Verification items for the finished model (mm, model axes). A direction names the side the tool comes from. Give positions to 0.01 mm unless a question says otherwise; leave off trailing zeros. Loops run counter-clockwise (first coordinate to the right, second up) from the corner with the lowest first, then second, coordinate; pieces in that order, holes last. Notation, with made-up numbers: M -27,-19 L 4,-19 A14 cw 4,1 Z; hole C -5,-8 d1. An arc over 180 degrees is marked long. Use a Markdown table: item, result.
from build123d import *

# Parameters (mm, degrees)
F1_DEPTH = 62.4
F4_DEPTH = 24.5
F5_W     = 19.0535837948
F5_H     = 11.2809054554
F5_H_2   = 2.8878487647
F6_DEPTH = 4.1


# Not quite as in the source:
# - a pattern or mirror of a feature is missing from the dataset's text; its kind, count and spacing are read off the source's solid


with BuildPart() as f1:
    # F0 (on Right) → F1 (new body)
    with BuildSketch(Plane.YZ):
        Polygon((24.6393419802, 87.7444967628), (5.7596671395, 54.6524040401), (5.7596671395, 37.0838306844), (49.7630737395, 15.9439614351), (358.1593094913, 15.9439614351), (388.9961540699, 31.0895591974), (388.9961540699, 87.2576609254), (339.3792808056, 93.3623313904), (64.8232772946, 93.3623313904), align=None)
    extrude(amount=F1_DEPTH)

    # F2: F1 across plane


with BuildPart() as f1_1:
    add(f1.part)
    add(f1.part.mirror(Plane.YZ))

    # F3 (on face) → F4 (cut)
    with BuildSketch(Plane.YZ.offset(62.4)):
        Polygon((59.2419728637, 15.9439614351), (127.3969262838, 15.9439614351), (127.3969262838, 41.5049567819), (110.9381020069, 60.795918107), (75.7007971406, 60.795918107), (59.2419728637, 41.5049567819), align=None)
        Polygon((230.519130826, 15.9439614351), (342.7896499634, 15.9439614351), (342.7896499634, 36.7200672626), (333.9802026749, 60.795918107), (241.1305308342, 60.795918107), (230.519130826, 41.8756008148), align=None)
    f4 = extrude(amount=-F4_DEPTH, mode=Mode.SUBTRACT)

    # F4_copies: F4 across plane
    add(f4.mirror(Plane(origin=(0, 0, 0), x_dir=(0, 0, -1), z_dir=(-1, 0, 0))), mode=Mode.SUBTRACT)

    # F5 (on face) → F6 (cut)
    with BuildSketch(Plane.XZ.offset(-5.7596671395)):
        with Locations((52.8732081026, 42.7242834121)):
            Rectangle(F5_W, F5_H)
        with Locations((52.8732081026, 35.6399063021)):
            Rectangle(F5_W, F5_H_2)
    f6 = extrude(amount=-F6_DEPTH, mode=Mode.SUBTRACT)

    # F6_copies: F6 across plane
    add(f6.mirror(Plane(origin=(0, 0, 0), x_dir=(0, 0, -1), z_dir=(-1, 0, 0))), mode=Mode.SUBTRACT)


solid = f1_1.part
(1) Cross-section at C-C on x = 51. Record the cut outline in (y, z).
Results below:
| item | result |
|---|---|
| outline | M 5.76,48.36 L 9.86,48.36 L 9.86,35.11 L 49.76,15.94 L 59.24,15.94 L 59.24,41.5 L 75.7,60.8 L 110.94,60.8 L 127.4,41.5 L 127.4,15.94 L 230.52,15.94 L 230.52,41.88 L 241.13,60.8 L 333.98,60.8 L 342.79,36.72 L 342.79,15.94 L 358.16,15.94 L 389,31.09 L 389,87.26 L 339.38,93.36 L 64.82,93.36 L 24.64,87.74 L 5.76,54.65 Z |
(2) Cross-section at A-A on y = 310.5. Record the cut outline in (x, z).
Results below:
| item | result |
|---|---|
| outline | M -62.4,60.8 L -37.9,60.8 L -37.9,15.94 L 37.9,15.94 L 37.9,60.8 L 62.4,60.8 L 62.4,93.36 L -62.4,93.36 Z |
(3) Material ranges on line 1 (Y direction, x = -51, z = 58); line 2 (Y direction, x = -51, z = 44); line 3 (X direction, y = 314, z = 43.5), recorded low to high.
Results below:
| item | result |
|---|---|
| line 1 | 7.67 to 73.32, 113.32 to 239.56, 335 to 389 |
| line 2 | 9.86 to 61.37, 125.27 to 231.71, 340.13 to 389 |
| line 3 | -37.9 to 37.9 |
(4) Cross-section at B-B on x = -18. Record the cut outline in (y, z), then the cut area to 3 significant figures.
Results below:
| item | result |
|---|---|
| outline | M 5.76,37.08 L 49.76,15.94 L 358.16,15.94 L 389,31.09 L 389,87.26 L 339.38,93.36 L 64.82,93.36 L 24.64,87.74 L 5.76,54.65 Z |
| area | 28,300 mm^2 |
(5) Set-up check for faces 5 (the flat face through (50, 288, 60.796)), 6 (the flat face through (-50, 288, 60.796)), 7 (the flat face through (1, 204, 93.362)): record each of +Z, -Z, +X, -X, +Y, -Y from which the full face is reachable in a straight line by a thin tool's end or side.
Results below:
| item | result |
|---|---|
| face 5 | -Z, +X |
| face 6 | -Z, -X |
| face 7 | +Z, +X, -X, +Y, -Y |
(6) Draft check along Y on faces 1 (the flat face through (50, 59.242, 29)), 2 (the flat face through (0.874, 364.535, 90.267)), 3 (the flat face through (-53, 9.86, 42)), 4 (the flat face through (62.4, 195, 64)). Enter one of: +Y half, -Y half, draft (parallel to the pull), parting line (faces both ways), or undercut.
Results below:
| item | result |
|---|---|
| face 1 | undercut |
| face 2 | +Y half |
| face 3 | -Y half |
| face 4 | draft |
(7) Cross-section at D-D on z = 70. Record the cut outline in (x, y), then the cut area to 3 significant figures.
Results below:
| item | result |
|---|---|
| outline | M -62.4,14.52 L 62.4,14.52 L 62.4,389 L -62.4,389 Z |
| area | 46,700 mm^2 |
(8) Gauge pin test, flat ends, axial feed: P1, Ø6, axis at x = -45.5, z = 85, coming from the -Y side; P2, Ø6, axis at x = -49, z = 76.5, coming from the -Y side; P3, Ø1.5, axis at y = 236, z = 46, coming from the -X side. Record the tip position at first contact, or that the pin passes through.
Results below:
| item | result |
|---|---|
| P1 | y = 21.36 |
| P2 | y = 16.51 |
| P3 | x = -37.9 |
